Work out the finished part from the listing and answer in its coordinate system (mm). Coordinates: 2 decimals unless noted, no trailing zeros. Write each loop counter-clockwise with the first axis right and the second up, starting at its lowest first coordinate (ties: lowest second). Pieces come first, ordered by that corner, then holes. Notation, with made-up numbers: (-30, 47.5) - (9, 47.5) arc R18 cw to (9, 62.5) - close; hole circle Ø3 at (43, 89.5). An arc over 180 degrees is marked (long way). One line per item, written item: value.
Autodesk Inventor part; units mm, degrees
ref_plane "YZ Plane" through (0, 0, 0) normal (1, 0, 0) x (0, 1, 0)
ref_plane "XZ Plane" through (0, 0, 0) normal (0, 1, 0) x (-1, 0, 0)
ref_plane "XY Plane" through (0, 0, 0) normal (0, 0, 1) x (1, 0, 0)
ref_plane "Work Plane1" through (0, 0, 0) normal (0, 0, 1) x (1, 0, 0)
sketch "Sketch1" plane through (0, 0, 0) normal (0, 0, 1) x (1, 0, 0)
  circle A0 centre (-51.5287, 16.3728) radius 1.397
  circle A1 centre (-33.9472, 20.9752) radius 1.397
  line L0 (-56.5305, 24.9164) -> (-45.777, -18.2132)
  line L1 (-22.1173, -12.3142) -> (-32.8708, 30.8155)
  line L2 (-55.9143, 25.0701) -> (-33.4869, 30.6618)
  line L3 (-32.7171, 30.1993) -> (-29.7982, 18.4919)
  line L4 (-53.4579, 12.5929) -> (-56.3768, 24.3003)
  circle A2 centre (-42.2695, 18.1155) radius 1.5875
  arc A3 (-37.6286, 19.1777) -> (-46.8891, 16.9637) centre (-42.2695, 18.1155) ccw
  line L5 (-42.2695, 18.1155) -> (-54.0994, 15.1659) construction
  line L6 (-46.8891, 16.9637) -> (-46.862, 16.8552)
  line L7 (-37.6509, 19.267) -> (-37.6238, 19.1585)
  line L8 (-30.2607, 17.7222) -> (-33.775, 16.8459)
  line L9 (-49.1746, 13.0064) -> (-52.6881, 12.1304)
  arc A4 (-49.1746, 13.0064) -> (-46.862, 16.8552) centre (-49.9427, 16.0871) ccw
  arc A5 (-37.6238, 19.1585) -> (-33.775, 16.8459) centre (-34.5431, 19.9266) ccw
  arc A6 (-55.9143, 25.0701) -> (-56.3768, 24.3003) centre (-55.7607, 24.4539) ccw
  arc A7 (-32.7171, 30.1993) -> (-33.4869, 30.6618) centre (-33.3333, 30.0457) ccw
  arc A8 (-53.4579, 12.5929) -> (-52.6881, 12.1304) centre (-52.8417, 12.7465) ccw
  arc A9 (-30.2607, 17.7222) -> (-29.7982, 18.4919) centre (-30.4143, 18.3383) ccw
  point P0 (0, 0)
  dimension "d0" = 3.175
  dimension "d1" = 0.635
  dimension "d2" = 0.635
extrude "Extrusion1" add sketch "Sketch1" along normal blind 3.175 contours A6 L2 A7 L1 A9 L8 A5 L7 A3 L6 A4 L9 A8 L0
properties part number "spacerBlock01" material "Wood (Maple)"
Item 1: Consider probe 1 along X at (y, z) = (21.25, 2.4); probe 2 along X at (y, z) = (16.25, 0.5); probe 3 along X at (y, z) = (13.25, 1). Determine where each line is inside the solid, lowest interval first.
Evaluation:
probe 1: x = -55.62 to -45.85, -38.69 to -35.32, -32.58 to -30.49
probe 2: x = -54.37 to -52.92, -50.14 to -46.77
probe 3: x = -53.62 to -48.52
Item 2: Given pin 1 (1.5 mm diameter, centred on x = -43, z = 1.5, fed in from -Y), flat-ended and moving along its own axis, determine where the tip first touches the part or whether it passes through.
Evaluation:
pin 1: stops at y = 22.64
Item 3: Section A-A, the plane y = 15.5 is taken. Determine the outline of the cut face in (x, z) (1 decimal), then the cut area to 3 significant figures.
Evaluation:
outline: (-54.2, 0) - (-52.6, 0) - (-52.6, 3.2) - (-54.2, 3.2) - close; (-50.4, 0) - (-46.8, 0) - (-46.8, 3.2) - (-50.4, 3.2) - close
area: 16.4 mm2
Item 4: Section C-C, the plane x = -38.75 is taken. Determine the outline of the cut face in (y, z) (3 decimals), then the cut area to 3 significant figures.
Evaluation:
outline: (21.322, 0) - (29.35, 0) - (29.35, 3.175) - (21.322, 3.175) - close
area: 25.5 mm2
Item 5: Section D-D, the plane y = 28.25 is taken. Determine the outline of the cut face in (x, z) (3 decimals), then the cut area to 3 significant figures.
Evaluation:
outline: (-43.16, 0) - (-32.231, 0) - (-32.231, 3.175) - (-43.16, 3.175) - close
area: 34.7 mm2
Item 6: Determine the mould class of faces 1 (the face through (-43, 24, 3.175)), 2 (the face through (-36.15, 17.19, 1.57)), 3 (the face through (-50.24, 16.91, 1.57)), 4 (the face through (-44.858, 27.827, 1.565)) for opening direction Y: +Y half, -Y half, draft (parallel to the pull), parting line (faces both ways), or undercut.
Evaluation:
face 1: draft
face 2: -Y half
face 3: undercut
face 4: +Y half
Item 7: Section B-B, the plane z = 1.55 is taken. Give the number of separate pieces and of enclosed holes in the cut face, then the cut area to 3 significant figures.
Evaluation:
separate pieces: 1
enclosed holes: 2
area: 241 mm2
